CAD build for the part. Positions are in the model's coordinates, mm. Coordinates: 2 decimals unless noted, no trailing zeros. Write each loop counter-clockwise with the first axis right and the second up, starting at its lowest first coordinate (ties: lowest second). Pieces come first, ordered by that corner, then holes. Notation, with made-up numbers: M 44.5,68 L 53.5,68 A16 cw 53.5,73 Z; hole C -29,81 d5. An arc over 180 degrees is marked long. Put each result on its own line as item: value. Start each with the question number.
```python
from build123d import *

# Parameters (mm, degrees)
BOSS_EXTRUDE1_DEPTH = 5
SKETCH2_R           = 2
CUT_EXTRUDE1_DEPTH  = 6


with BuildPart() as part:
    # Sketch1 → Boss-Extrude1 (new body)
    with BuildSketch(Plane(origin=(0, 329.925662842, 0), x_dir=(1, 0, 0), z_dir=(0, 1, 0))):
        Polygon((507.724872759, 70.717280325), (507.724872759, 45.317280325), (565.699872759, 45.317280325), (565.699872759, -503.882719675), (507.724872759, -503.882719675), (507.724872759, -529.282719675), (344.299872759, -529.282719675), (344.299872759, -396.017719675), (196.299872759, -396.017719675), (196.299872759, -529.282719675), (32.874872759, -529.282719675), (32.874872759, -503.882719675), (-25.100127241, -503.882719675), (-21.925127241, 45.317280325), (32.874872759, 45.317280325), (32.874872759, 70.717280325), align=None)
    extrude(amount=BOSS_EXTRUDE1_DEPTH)

    # Sketch2 → Cut-Extrude1 (cut, through all)
    with BuildSketch(Plane.XZ.offset(-329.925662842)):
        with Locations((60.299872759, 518.607719675)):
            Circle(SKETCH2_R)
        with Locations((380.299872759, 518.607719675)):
            Circle(SKETCH2_R)
        with Locations((220.299872759, -60.042280325)):
            Circle(SKETCH2_R)
        with Locations((100.299872759, 518.607719675)):
            Circle(SKETCH2_R)
        with Locations((420.299872759, 518.607719675)):
            Circle(SKETCH2_R)
        with Locations((260.299872759, -60.042280325)):
            Circle(SKETCH2_R)
        with Locations((140.299872759, 518.607719675)):
            Circle(SKETCH2_R)
        with Locations((460.299872759, 518.607719675)):
            Circle(SKETCH2_R)
        with Locations((300.299872759, -60.042280325)):
            Circle(SKETCH2_R)
        with Locations((180.299872759, 518.607719675)):
            Circle(SKETCH2_R)
        with Locations((500.299872759, 518.607719675)):
            Circle(SKETCH2_R)
        with Locations((340.299872759, -60.042280325)):
            Circle(SKETCH2_R)
        with Locations((-14.425127241, 239.282719675)):
            Circle(SKETCH2_R)
        with Locations((555.024872759, 239.282719675)):
            Circle(SKETCH2_R)
        with Locations((-14.425127241, 279.282719675)):
            Circle(SKETCH2_R)
        with Locations((555.024872759, 279.282719675)):
            Circle(SKETCH2_R)
        with Locations((-14.425127241, 319.282719675)):
            Circle(SKETCH2_R)
        with Locations((555.024872759, 319.282719675)):
            Circle(SKETCH2_R)
        with Locations((-14.425127241, 359.282719675)):
            Circle(SKETCH2_R)
        with Locations((555.024872759, 359.282719675)):
            Circle(SKETCH2_R)
        with Locations((-14.425127241, 399.282719675)):
            Circle(SKETCH2_R)
        with Locations((555.024872759, 399.282719675)):
            Circle(SKETCH2_R)
        with Locations((-14.425127241, 439.282719675)):
            Circle(SKETCH2_R)
        with Locations((555.024872759, 439.282719675)):
            Circle(SKETCH2_R)
        with Locations((-14.425127241, 479.282719675)):
            Circle(SKETCH2_R)
        with Locations((555.024872759, 479.282719675)):
            Circle(SKETCH2_R)
    extrude(amount=-CUT_EXTRUDE1_DEPTH, mode=Mode.SUBTRACT)


solid = part.part
```
(1) Slice it at B-B, the plane x = 240.5. Write the cut outline in (y, z), then the cut area to 3 significant figures.
(2) Drop flat-ended pins along their axis: pin 1 (1.5 mm diameter, centred on x = 523, y = 333.5, fed in from -Z); pin 2 (2.5 mm diameter, centred on x = 547, y = 333, fed in from +Z); pin 3 (1 mm diameter, centred on y = 333.5, z = 85.5, fed in from -X). Give the stop position or say it passes through.
(3) Drill centre lines: line 1 (X direction, y = 334.1, z = 441); line 2 (X direction, y = 330.5, z = 477.5); line 3 (X direction, y = 330.7, z = 321). Where is each one in solid material? Low to high. Write a range as [from, to].
(4) Slice it at A-A, the plane y = 330.7. State how many separate pieces and enclosed holes the cut face has, then the cut area to 3 significant figures.
Result set:
1. outline: M 329.93,-70.72 L 334.93,-70.72 L 334.93,396.02 L 329.93,396.02 Z
1. area: 2,330 mm^2
2. pin 1: stops at z = -45.32
2. pin 2: stops at z = 503.88
2. pin 3: stops at x = -22.68
3. line 1: x = [-24.74, -15.45], [-13.4, 196.3], [344.3, 554], [556.05, 565.7]
3. line 2: x = [-24.95, -15.33], [-13.52, 196.3], [344.3, 554.12], [555.93, 565.7]
3. line 3: x = [-24.04, -15.45], [-13.4, 554], [556.05, 565.7]
4. separate pieces: 1
4. enclosed holes: 26
4. area: 328,000 mm^2
